Source: CAD feature listing. Evaluate the final solid. Frame: model axes, mm. A direction names the side the tool comes from. Give positions to 0.01 mm unless a question says otherwise; leave off trailing zeros. Loops run counter-clockwise (first coordinate to the right, second up) from the corner with the lowest first, then second, coordinate; pieces in that order, holes last. Notation, with made-up numbers: (8, 32) -> (45, 32) arc R20 cw to (45, 56) -> close; hole circle Ø11 at (54, 2.5). An arc over 180 degrees is marked (long way). Return JSON: item names as keys, results as strings. Group by question number.
(1) Pin query (flat end, axial travel): pin 1 (7 mm diameter, centred on y = -22, z = -4, fed in from -X); pin 2 (9 mm diameter, centred on x = 0, y = 0, fed in from -Z); pin 3 (10 mm diameter, centred on y = -13, z = -3.5, fed in from -X). Return the tip coordinate at first contact, or that it passes through.
(2) Cut plane A-A on z = 4. Return loops of the section in (x, y), then the cut area to 3 significant figures.
(3) Cut plane C-C on z = -17.7. Return loops of the section in (x, y), then the cut area to 3 significant figures.
(4) Ray query, line 1 (Y direction, x = 0, z = 6); line 2 (Z direction, x = 0, y = -25.4); line 3 (Z direction, x = 3, y = 8). Return the intervals inside material, ascending. Write a range as from..to.
(5) Access query for faces 1 (the face through (0.595, -26.056, -18.156)), 2 (the face through (4, -25, -4)), 3 (the face through (-4, -25, -4)). Directions: +Z, -Z, +X, -X, +Y, -Y. A direction counts if a zero-diameter tool reaches every point of the face in a straight line with its end or side. Return the directions, or none.
(6) Cut plane B-B on x = 0. Return loops of the section in (y, z).
(7) Cut plane D-D on x = 9.15. Return loops of the section in (y, z).
(8) Draft query along Y for faces 4 (the face through (9.865, -0.225, 4.437)), 5 (the face through (0, -24.084, -12)), 6 (the face through (4, -2, 0)). Return one class per face: released by +Y, released by -Y, zero draft, split by the parting line, or undercut.
```python
from build123d import *

# Parameters (mm, degrees)
F0_R      = 19.5
F1_DEPTH  = 9
F2_R      = 2.85
F3_DEPTH  = 9.001
F4_W      = 8
F4_H      = 9
F5_DEPTH  = 9
F6_W      = 8
F6_H      = 4
F7_DEPTH  = 24
F8_R      = 0.75
F9_DEPTH  = 9.001
F10_R     = 0.75
F11_DEPTH = 4.001


with BuildPart() as f1:
    # F0 (on Top) → F1 (new body)
    with BuildSketch(Plane.XY):
        Circle(F0_R)
    extrude(amount=F1_DEPTH)

    # F2 (on face) → F3 (cut, through all)
    with BuildSketch(Plane.XY.offset(9)):
        Circle(F2_R)
    extrude(amount=-F3_DEPTH, mode=Mode.SUBTRACT)

    # F4 (on face) → F5 (join)
    with BuildSketch(Plane(origin=(0, 0, 0), x_dir=(1, 0, 0), z_dir=(0, 0, -1))):
        with Locations((0, 23.583922)):
            Rectangle(F4_W, F4_H)
    extrude(amount=-F5_DEPTH)

    # F6 (on face) → F7 (join)
    with BuildSketch(Plane(origin=(0, 0, 0), x_dir=(1, 0, 0), z_dir=(0, 0, -1))):
        with Locations((0, 26.083922)):
            Rectangle(F6_W, F6_H)
    extrude(amount=F7_DEPTH)

    # F8 (on face) → F9 (cut, through all)
    with BuildSketch(Plane(origin=(0, 0, 0), x_dir=(1, 0, 0), z_dir=(0, 0, -1))):
        with Locations((-9.15, 0)):
            Circle(F8_R)
        with Locations((9.15, 0)):
            Circle(F8_R)
    extrude(amount=-F9_DEPTH, mode=Mode.SUBTRACT)

    # F10 (on face) → F11 (cut, through all)
    with BuildSketch(Plane(origin=(0, -24.083922, 0), x_dir=(-1, 0, 0), z_dir=(0, 1, 0))):
        with Locations((0, -17.7)):
            Circle(F10_R)
    extrude(amount=-F11_DEPTH, mode=Mode.SUBTRACT)


solid = f1.part
```
Answers:
{
 "1": {"pin 1": "x = -4", "pin 2": "z = 0", "pin 3": "x = -17.07"},
 "2": {"outline": "(-4, -28.08) -> (4, -28.08) -> (4, -19.09) arc R19.5 ccw (long way) to (-4, -19.09) -> close; hole circle Ø1.5 at (-9.15, 0); hole circle Ø5.7 at (0, 0); hole circle Ø1.5 at (9.15, 0)", "area": "1,240 mm²"},
 "3": {"outline": "(-4, -28.08) -> (-0.75, -28.08) -> (-0.75, -24.08) -> (-4, -24.08) -> close; (0.75, -28.08) -> (4, -28.08) -> (4, -24.08) -> (0.75, -24.08) -> close", "area": "26.0 mm²"},
 "4": {"line 1": "-28.08..-2.85, 2.85..19.5", "line 2": "-24..-18.45, -16.95..9", "line 3": "0..9"},
 "5": {"face 1": "+Y, -Y", "face 2": "+Z, -Z, +X, -Y", "face 3": "+Z, -Z, -X, -Y"},
 "6": {"outline": "(-28.08, -24) -> (-24.08, -24) -> (-24.08, -18.45) -> (-28.08, -18.45) -> close; (-28.08, -16.95) -> (-24.08, -16.95) -> (-24.08, 0) -> (-2.85, 0) -> (-2.85, 9) -> (-28.08, 9) -> close; (2.85, 0) -> (19.5, 0) -> (19.5, 9) -> (2.85, 9) -> close"},
 "7": {"outline": "(-17.22, 0) -> (-0.75, 0) -> (-0.75, 9) -> (-17.22, 9) -> close; (0.75, 0) -> (17.22, 0) -> (17.22, 9) -> (0.75, 9) -> close"},
 "8": {"face 4": "undercut", "face 5": "released by +Y", "face 6": "zero draft"}
}
